Geometry: final body of the model. Coordinates: model frame, mm. A direction names the side the tool comes from. Coordinates: 2 decimals unless noted, no trailing zeros. Write each loop counter-clockwise with the first axis right and the second up, starting at its lowest first coordinate (ties: lowest second). Pieces come first, ordered by that corner, then holes. Notation, with made-up numbers: (18.5, 44) -> (42.5, 44) arc R20 cw to (42.5, 48) -> close; hole circle Ø2 at (47, 66.5). An arc over 180 degrees is marked (long way). One line per item, written item: value.
```python
from build123d import *

# Parameters (mm, degrees)
PAD_DEPTH            = 87
SKETCH001_R          = 4.165
POCKET_DEPTH         = 0.001
POCKET_DEPTH_BACK    = 45.001
SKETCH002_R          = 4.165
POCKET001_DEPTH      = 0.001
POCKET001_DEPTH_BACK = 45.001
FILLET_R             = 5
SKETCH004_R          = 2.38125
POCKET002_DEPTH      = 0.001
POCKET002_DEPTH_BACK = 45.001
LINEARPATTERN_COUNT  = 2
LINEARPATTERN_PITCH  = 45
SKETCH005_R          = 5.55625
SKETCH005_R_2        = 1.867
POCKET003_DEPTH      = 0.001
POCKET003_DEPTH_BACK = 45.001
SKETCH006_R          = 1.45
HOLE_DEPTH           = 10
HOLE_TIPS_R          = 1.45
SKETCH007_W          = 60
SKETCH007_H          = 60
POCKET004_DEPTH      = 43.5


with BuildPart() as part:
    # Sketch → Pad (new body)
    with BuildSketch(Plane.XY):
        Polygon((0, 0), (45, 0), (45, -6), (6, -6), (6, -45), (0, -45), align=None)
    extrude(amount=PAD_DEPTH)

    # Sketch001 → Pocket (cut, two sides)
    with BuildSketch(Plane.YZ) as pocket_sk:
        with Locations((-22.5, 21)):
            Circle(SKETCH001_R)
        with Locations((-22.5, 66)):
            Circle(SKETCH001_R)
    extrude(amount=-POCKET_DEPTH, mode=Mode.SUBTRACT)
    extrude(pocket_sk.sketch, amount=POCKET_DEPTH_BACK, mode=Mode.SUBTRACT)

    # Sketch002 → Pocket001 (cut, two sides)
    with BuildSketch(Plane.XZ) as pocket001_sk:
        with Locations((22.5, 66)):
            Circle(SKETCH002_R)
        with Locations((22.5, 21)):
            Circle(SKETCH002_R)
    extrude(amount=-POCKET001_DEPTH, mode=Mode.SUBTRACT)
    extrude(pocket001_sk.sketch, amount=POCKET001_DEPTH_BACK, mode=Mode.SUBTRACT)

    # Fillet
    fillet_edges = [part.edges().sort_by_distance(p)[0] for p in [
        (6, -45, 43.5),
        (45, -6, 43.5),
        (6, -6, 43.5),
    ]]
    fillet(fillet_edges, radius=FILLET_R)

    # Sketch004 → Pocket002 (cut, two sides)
    with BuildSketch(Plane.YZ) as pocket002_sk:
        with Locations((-14.5625, 21)):
            Circle(SKETCH004_R)
        with Locations((-30.4375, 21)):
            Circle(SKETCH004_R)
    pocket002 = extrude(amount=-POCKET002_DEPTH, mode=Mode.SUBTRACT) + extrude(pocket002_sk.sketch, amount=POCKET002_DEPTH_BACK, mode=Mode.SUBTRACT)

    # LinearPattern: Pocket002 ×2
    with Locations(*[(0, 0, i * LINEARPATTERN_PITCH) for i in range(1, LINEARPATTERN_COUNT)]):
        add(pocket002, mode=Mode.SUBTRACT)

    # Sketch005 → Pocket003 (cut, two sides)
    with BuildSketch(Plane.YZ) as pocket003_sk:
        with Locations((-22.5, 43.5)):
            Circle(SKETCH005_R)
        with Locations((-28.156854, 49.156854)):
            Circle(SKETCH005_R_2)
        with Locations((-16.843146, 37.843146)):
            Circle(SKETCH005_R_2)
        with Locations((-16.843146, 49.156854)):
            Circle(SKETCH005_R_2)
        with Locations((-28.156854, 37.843146)):
            Circle(SKETCH005_R_2)
    extrude(amount=-POCKET003_DEPTH, mode=Mode.SUBTRACT)
    extrude(pocket003_sk.sketch, amount=POCKET003_DEPTH_BACK, mode=Mode.SUBTRACT)

    # Sketch006 → Hole (cut)
    with BuildSketch(Plane.XZ):
        with Locations((7, 81.5)):
            Circle(SKETCH006_R)
        with Locations((38, 81.5)):
            Circle(SKETCH006_R)
        with Locations((38, 50.5)):
            Circle(SKETCH006_R)
        with Locations((7, 50.5)):
            Circle(SKETCH006_R)
    extrude(amount=HOLE_DEPTH, mode=Mode.SUBTRACT)

    # Hole tips → Hole tip 1 section 0
    with BuildSketch(Plane.XZ.offset(10), mode=Mode.PRIVATE) as hole_tip_1_s0:
        with Locations((7, 81.5)):
            Circle(HOLE_TIPS_R)
    loft([hole_tip_1_s0.sketch, Vertex(7, -10.871248, 81.5)], mode=Mode.SUBTRACT)

    # Hole tips → Hole tip 2 section 0
    with BuildSketch(Plane.XZ.offset(10), mode=Mode.PRIVATE) as hole_tip_2_s0:
        with Locations((38, 81.5)):
            Circle(HOLE_TIPS_R)
    loft([hole_tip_2_s0.sketch, Vertex(38, -10.871248, 81.5)], mode=Mode.SUBTRACT)

    # Hole tips → Hole tip 3 section 0
    with BuildSketch(Plane.XZ.offset(10), mode=Mode.PRIVATE) as hole_tip_3_s0:
        with Locations((38, 50.5)):
            Circle(HOLE_TIPS_R)
    loft([hole_tip_3_s0.sketch, Vertex(38, -10.871248, 50.5)], mode=Mode.SUBTRACT)

    # Hole tips → Hole tip 4 section 0
    with BuildSketch(Plane.XZ.offset(10), mode=Mode.PRIVATE) as hole_tip_4_s0:
        with Locations((7, 50.5)):
            Circle(HOLE_TIPS_R)
    loft([hole_tip_4_s0.sketch, Vertex(7, -10.871248, 50.5)], mode=Mode.SUBTRACT)

    # Sketch007 → Pocket004 (cut)
    with BuildSketch(Plane.XY):
        with Locations((36, 0)):
            Rectangle(SKETCH007_W, SKETCH007_H)
    extrude(amount=POCKET004_DEPTH, mode=Mode.SUBTRACT)


solid = part.part
```
(1) First-contact query: pin 1 (5 mm diameter, centred on y = -16.84, z = 49.16, fed in from +X); pin 2 (9 mm diameter, centred on x = 30.5, y = -3.5, fed in from -Z); pin 3 (8.5 mm diameter, centred on x = 31.5, z = 76, fed in from -Y). Flat tips, straight axial feed; report the tip coordinate or a pass-through.
Responses:
pin 1: stops at x = 6
pin 2: stops at z = 43.5
pin 3: stops at y = -6
(2) Section D-D (z = 66). Return the cut outline in (x, y) (3 decimals).
Responses:
outline: (0, -45) -> (1, -45) arc R5 ccw to (6, -40) -> (6, -32.819) -> (0, -32.819) -> close; (0, -28.056) -> (6, -28.056) -> (6, -26.665) -> (0, -26.665) -> close; (0, -18.335) -> (6, -18.335) -> (6, -16.944) -> (0, -16.944) -> close; (0, -12.181) -> (6, -12.181) -> (6, -11) arc R5 cw to (11, -6) -> (18.335, -6) -> (18.335, 0) -> (0, 0) -> close; (26.665, -6) -> (40, -6) arc R5 ccw to (45, -1) -> (45, 0) -> (26.665, 0) -> close
(3) Pull-direction query (X, two-part tool) for faces 1 (the cylindrical face through (36.55, -2.96, 50.56)), 2 (the flat face through (0, -23, 33)), 3 (the cylindrical face through (24.74, -2.96, 69.51)), 4 (the flat face through (3, -22, 0)); classes: released by +X, released by -X, zero draft, split by the parting line, or undercut.
Responses:
face 1: undercut
face 2: released by -X
face 3: undercut
face 4: zero draft
(4) Section C-C (y = -22.5). Return the cut outline in (x, z) (3 decimals), then the cut area to 3 significant figures.
Responses:
outline: (0, 0) -> (6, 0) -> (6, 16.835) -> (0, 16.835) -> close; (0, 25.165) -> (6, 25.165) -> (6, 37.944) -> (0, 37.944) -> close; (0, 49.056) -> (6, 49.056) -> (6, 61.835) -> (0, 61.835) -> close; (0, 70.165) -> (6, 70.165) -> (6, 87) -> (0, 87) -> close
area: 355 mm2
(5) Reachability of faces 5 (the flat face through (6, -24, 33)), 6 (the cylindrical face through (5.55, -3.82, 81.56)), 7 (the flat face through (29, -6, 65)), 8 (the flat face through (25, -3, 43.5)) from +Z, -Z, +X, -X, +Y, -Y: full face, straight path, thin tool, end or side. Return the list, or none.
Responses:
face 5: -Z, +X, -Y
face 6: +Y
face 7: +Z, -Z, +X, -Y
face 8: -Z, +X, +Y, -Y
(6) Section B-B (x = 7). Return the cut outline in (y, z).
Responses:
outline: (-8, 43.5) -> (0, 43.5) -> (0, 49.05) -> (-8, 49.05) -> close; (-8, 51.95) -> (0, 51.95) -> (0, 80.05) -> (-8, 80.05) -> close; (-8, 82.95) -> (0, 82.95) -> (0, 87) -> (-8, 87) -> close
(7) Section A-A (z = 21). Return the cut outline in (x, y) (3 decimals), then the cut area to 3 significant figures.
Responses:
outline: (0, -45) -> (1, -45) arc R5 ccw to (6, -40) -> (6, -32.819) -> (0, -32.819) -> close; (0, -28.056) -> (6, -28.056) -> (6, -26.665) -> (0, -26.665) -> close; (0, -18.335) -> (6, -18.335) -> (6, -16.944) -> (0, -16.944) -> close; (0, -12.181) -> (6, -12.181) -> (6, 0) -> (0, 0) -> close
area: 158 mm2
(8) Line query: line 1 (Z direction, x = 7, y = -4.25); line 2 (X direction, y = -1, z = 66) (3 decimals); line 3 (X direction, y = -21, z = 7.5). Output: solid intervals per line, ascending. Write a range as [from, to].
Responses:
line 1: z = [43.5, 49.05], [51.95, 80.05], [82.95, 87]
line 2: x = [0, 18.335], [26.665, 45]
line 3: x = [0, 6]
